```python
from build123d import *

# Parameters (mm, degrees)
SKETCH_1_W               = 65
SKETCH_1_H               = 92
SKETCH_1_W_2             = 59
SKETCH_1_H_2             = 86
EXTRUDE_1_DEPTH          = 26
SKETCH_2_W               = 65
SKETCH_2_H               = 105
EXTRUDE_2_DEPTH          = 3
CUT_EXTRUDE_1_DEPTH      = 67.996268553
CUT_EXTRUDE_1_DEPTH_BACK = 67.996268553
SKETCH_3_R               = 1.6
FILLET_1_R               = 3
CUT_EXTRUDE_START        = -3
CUT_EXTRUDE_2_OUTLINE_W  = 14
CUT_EXTRUDE_2_OUTLINE_H  = 10
CUT_EXTRUDE_2_DEPTH      = 3
CUT_EXTRUDE_3_OUTLINE_W  = 10
CUT_EXTRUDE_3_OUTLINE_H  = 11
CUT_EXTRUDE_3_DEPTH      = 3
SKETCH_6_W               = 14
SKETCH_6_H               = 6
CUT_EXTRUDE_4_DEPTH      = 10


# Read off the part's stored shape, not the designer's step: 切除-拉伸2, 切除-拉伸3
with BuildPart() as part:
    # 草图1 → 凸台-拉伸1 (new body)
    with BuildSketch(Plane(origin=(0, 0, 0), x_dir=(1, 0, 0), z_dir=(0, 1, 0))):
        Rectangle(SKETCH_1_W, SKETCH_1_H)
        Rectangle(SKETCH_1_W_2, SKETCH_1_H_2, mode=Mode.SUBTRACT)
    extrude(amount=EXTRUDE_1_DEPTH)

    # 草图2 → 凸台-拉伸2 (add)
    with BuildSketch(Plane.XZ):
        Rectangle(SKETCH_2_W, SKETCH_2_H)
    extrude(amount=EXTRUDE_2_DEPTH)

    # 草图3 → 切除-拉伸1 (cut, two sides: drawn at the far end of the back side and taken through both)
    with BuildSketch(Plane(origin=(0, 0, 0), x_dir=(1, 0, 0), z_dir=(0, 1, 0)).offset(-CUT_EXTRUDE_1_DEPTH_BACK)):
        with Locations(Location((-26, 49.5, 0), (0, 0, 270))):
            Circle(SKETCH_3_R)
        with Locations(Location((26, 49.5, 0), (0, 0, 270))):
            Circle(SKETCH_3_R)
        with Locations(Location((26, -49.5, 0), (0, 0, 270))):
            Circle(SKETCH_3_R)
        with Locations(Location((-26, -49.5, 0), (0, 0, 270))):
            Circle(SKETCH_3_R)
    extrude(amount=CUT_EXTRUDE_1_DEPTH + CUT_EXTRUDE_1_DEPTH_BACK, mode=Mode.SUBTRACT)

    # 圆角1
    fillet_1_edges = [part.edges().sort_by_distance(p)[0] for p in [
        (32.5, -1.5, -52.5),
        (32.5, -1.5, 52.5),
        (-32.5, -1.5, 52.5),
        (-32.5, -1.5, -52.5),
    ]]
    fillet(fillet_1_edges, radius=FILLET_1_R)

    # 切除-拉伸2 outline → 切除-拉伸2 (cut)
    with BuildSketch(Plane(origin=(0, 0, 43), x_dir=(-1, 0, 0), z_dir=(0, 0, -1)).offset(CUT_EXTRUDE_START)):
        with Locations((0.5, 5)):
            Rectangle(CUT_EXTRUDE_2_OUTLINE_W, CUT_EXTRUDE_2_OUTLINE_H)
    extrude(amount=CUT_EXTRUDE_2_DEPTH, mode=Mode.SUBTRACT)

    # 切除-拉伸3 outline → 切除-拉伸3 (cut)
    with BuildSketch(Plane(origin=(-29.5, 0, 0), x_dir=(0, 0, -1), z_dir=(1, 0, 0)).offset(CUT_EXTRUDE_START)):
        with Locations((-28, 7.5)):
            Rectangle(CUT_EXTRUDE_3_OUTLINE_W, CUT_EXTRUDE_3_OUTLINE_H)
    extrude(amount=CUT_EXTRUDE_3_DEPTH, mode=Mode.SUBTRACT)

    # 草图6 → 切除-拉伸4 (cut)
    with BuildSketch(Plane(origin=(0, 0, -46), x_dir=(-1, 0, 0), z_dir=(0, 0, -1))):
        with Locations((0, 23)):
            Rectangle(SKETCH_6_W, SKETCH_6_H)
    extrude(amount=-CUT_EXTRUDE_4_DEPTH, mode=Mode.SUBTRACT)


solid = part.part
```
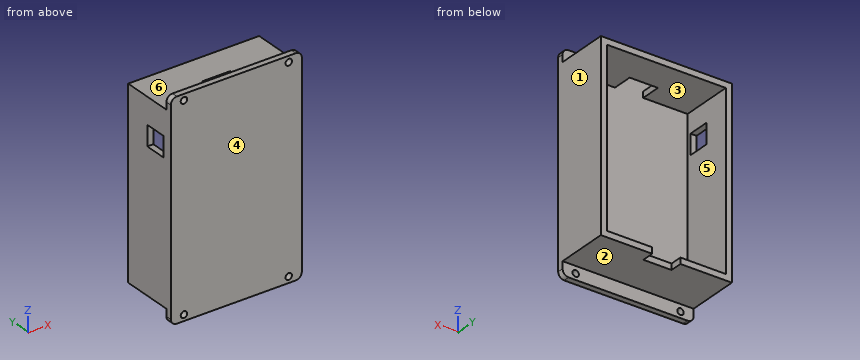
CAD build for the part. Positions are in the model's coordinates, mm. Face numbers are marked on the shaded views. A direction names the side the tool comes from. Round coordinates to 2 decimals unless told otherwise and drop trailing zeros. Write each loop counter-clockwise with the first axis right and the second up, starting at its lowest first coordinate (ties: lowest second). Pieces come first, ordered by that corner, then holes. Notation, with made-up numbers: (39, -2.5) -> (94, -2.5) arc R20 cw to (94, 4.5) -> close; hole circle Ø4 at (-30, -32). An arc over 180 degrees is marked (long way). Answer in a Markdown table with one row per item. Add a question column.
Item 1: Drop flat-ended pins along their axis: pin 1 Ø1 at (x, y) = (-3, 10.5) entering from -Z; pin 2 Ø0.9 at (x, z) = (1.5, -44.5) entering from +Y; pin 3 Ø5 at (x, z) = (26, -49.5) entering from +Y. Give the stop position or say it passes through.
Item 2: Mould opens along X. For the marked faces 1, 2 and 3 say: pulls with the +X half, pulls with the -X half, needs draft (parallel to the pull), parting line crosses it, or undercut.
Item 3: Saw through at D-D, the plane z = -40.5. Write the cut outline in (x, y), then the cut area to 3 significant figures.
Item 4: Which spindle directions (+Z, -Z, +X, -X, +Y, -Y) get a long thin tool onto all of the face, cutting with end or side? Do the marked faces 4, 5 and 6. Say none if no direction does.
Item 5: Saw through at C-C, the plane x = -26. Write the cut outline in (y, z), then the cut area to 3 significant figures.
Item 6: Drill centre lines: line 1 (X direction, y = -1.85, z = 49.5); line 2 (Z direction, x = 26, y = -1.95); line 3 (Z direction, x = -23.5, y = 3.5). Where is each one in solid material? Low to high. Write a range as from..to.
Item 7: Saw through at B-B, the plane y = 4.75. Write the cut outline in (x, z), then the cut area to 3 significant figures.
Item 8: Saw through at A-A, the plane x = 3. Write the cut outline in (y, z).
Findings below:
| question | item | result |
|---|---|---|
| 1 | pin 1 | stops at z = -46 |
| 1 | pin 2 | stops at y = 20 |
| 1 | pin 3 | stops at y = 0 |
| 2 | face 1 | pulls with the +X half |
| 2 | face 2 | needs draft |
| 2 | face 3 | undercut |
| 3 | outline | (-32.5, -3) -> (32.5, -3) -> (32.5, 26) -> (29.5, 26) -> (29.5, 0) -> (-29.5, 0) -> (-29.5, 26) -> (-32.5, 26) -> close |
| 3 | area | 351 mm^2 |
| 4 | face 4 | +Z, -Z, +X, -X, -Y |
| 4 | face 5 | +Y |
| 4 | face 6 | +Z, +X, -X, +Y |
| 5 | outline | (-3, -52.5) -> (0, -52.5) -> (0, -51.1) -> (-3, -51.1) -> close; (-3, -47.9) -> (0, -47.9) -> (0, -46) -> (26, -46) -> (26, -43) -> (0, -43) -> (0, 43) -> (26, 43) -> (26, 46) -> (0, 46) -> (0, 47.9) -> (-3, 47.9) -> close; (-3, 51.1) -> (0, 51.1) -> (0, 52.5) -> (-3, 52.5) -> close |
| 5 | area | 452 mm^2 |
| 6 | line 1 | x = -32.5..-27.6, -24.4..24.4, 27.6..32.5 |
| 6 | line 2 | z = -52.5..-51.1, -47.9..47.9, 51.1..52.5 |
| 6 | line 3 | z = -46..-43, 43..46 |
| 7 | outline | (-32.5, -46) -> (32.5, -46) -> (32.5, 46) -> (6.5, 46) -> (6.5, 43) -> (29.5, 43) -> (29.5, -43) -> (-29.5, -43) -> (-29.5, 23) -> (-32.5, 23) -> close; (-32.5, 33) -> (-29.5, 33) -> (-29.5, 43) -> (-7.5, 43) -> (-7.5, 46) -> (-32.5, 46) -> close |
| 7 | area | 834 mm^2 |
| 8 | outline | (-3, -52.5) -> (0, -52.5) -> (0, -46) -> (20, -46) -> (20, -43) -> (0, -43) -> (0, 52.5) -> (-3, 52.5) -> close; (10, 43) -> (26, 43) -> (26, 46) -> (10, 46) -> close |
